```python
from build123d import *

# Parameters (mm, degrees)
BOSS_EXTRUDE1_DEPTH = 4.064
CUT_EXTRUDE1_DEPTH  = 5.08


with BuildPart() as part:
    # Sketch1 → Boss-Extrude1 (new body)
    with BuildSketch(Plane.XY):
        Polygon((-223.0755, -19.05), (-219.0115, -19.05), (-219.0115, -31.75), (-223.0755, -31.75), (-223.0755, -95.25), (-219.0115, -95.25), (-219.0115, -107.95), (-223.0755, -107.95), (-223.0755, -120.65), (223.0755, -120.65), (223.0755, -107.95), (219.0115, -107.95), (219.0115, -95.25), (223.0755, -95.25), (223.0755, -31.75), (219.0115, -31.75), (219.0115, -19.05), (223.0755, -19.05), (223.0755, 0), (172.2755, 0), (172.2755, 4.064), (146.8755, 4.064), (146.8755, 0), (-146.8755, 0), (-146.8755, 4.064), (-172.2755, 4.064), (-172.2755, 0), (-223.0755, 0), align=None)
    extrude(amount=BOSS_EXTRUDE1_DEPTH)

    # Sketch2 → Cut-Extrude1 (cut)
    with BuildSketch(Plane.XY.offset(4.064)):
        with BuildLine():
            Line((-105.7275, -25.4), (105.7275, -25.4))
            ThreePointArc((105.7275, -25.4), (114.707756121, -29.119743879), (118.4275, -38.1))
            Line((118.4275, -38.1), (118.4275, -82.55))
            ThreePointArc((118.4275, -82.55), (114.707756121, -91.530256121), (105.7275, -95.25))
            Line((105.7275, -95.25), (-105.7275, -95.25))
            ThreePointArc((-105.7275, -95.25), (-114.707756121, -91.530256121), (-118.4275, -82.55))
            Line((-118.4275, -82.55), (-118.4275, -38.1))
            ThreePointArc((-118.4275, -38.1), (-114.707756121, -29.119743879), (-105.7275, -25.4))
        make_face()
        with BuildLine():
            Line((137.88887808, -72.091607461), (157.460892539, -91.66362192))
            ThreePointArc((157.460892539, -91.66362192), (160.154969375, -91.66362192), (160.154969375, -88.969545084))
            Line((160.154969375, -88.969545084), (140.582954916, -69.397530625))
            ThreePointArc((140.582954916, -69.397530625), (137.88887808, -69.397530625), (137.88887808, -72.091607461))
        make_face()
        with BuildLine():
            Line((175.064666479, -90.408858006), (139.143641994, -54.487833521))
            ThreePointArc((139.143641994, -54.487833521), (136.449565158, -54.487833521), (136.449565158, -57.181910358))
            Line((136.449565158, -57.181910358), (172.370589642, -93.102934842))
            ThreePointArc((172.370589642, -93.102934842), (175.064666479, -93.102934842), (175.064666479, -90.408858006))
        make_face()
        with BuildLine():
            Line((139.728723609, -46.990684627), (182.561815373, -89.823776391))
            ThreePointArc((182.561815373, -89.823776391), (185.255892209, -89.823776391), (185.255892209, -87.129699554))
            Line((185.255892209, -87.129699554), (142.422800446, -44.296607791))
            ThreePointArc((142.422800446, -44.296607791), (139.728723609, -44.296607791), (139.728723609, -46.990684627))
        make_face()
        with BuildLine():
            Line((145.429821279, -39.221398115), (190.331101885, -84.122678721))
            ThreePointArc((190.331101885, -84.122678721), (193.025178721, -84.122678721), (193.025178721, -81.428601885))
            Line((193.025178721, -81.428601885), (148.123898115, -36.527321279))
            ThreePointArc((148.123898115, -36.527321279), (145.429821279, -36.527321279), (145.429821279, -39.221398115))
        make_face()
        with BuildLine():
            Line((153.199107791, -33.520300446), (196.032199554, -76.353392209))
            ThreePointArc((196.032199554, -76.353392209), (198.726276391, -76.353392209), (198.726276391, -73.659315373))
            Line((198.726276391, -73.659315373), (155.893184627, -30.826223609))
            ThreePointArc((155.893184627, -30.826223609), (153.199107791, -30.826223609), (153.199107791, -33.520300446))
        make_face()
        with BuildLine():
            Line((202.005434842, -63.468089642), (166.084410358, -27.547065158))
            ThreePointArc((166.084410358, -27.547065158), (163.390333521, -27.547065158), (163.390333521, -30.241141994))
            Line((163.390333521, -30.241141994), (199.311358006, -66.162166479))
            ThreePointArc((199.311358006, -66.162166479), (202.005434842, -66.162166479), (202.005434842, -63.468089642))
        make_face()
        with BuildLine():
            Line((178.300030625, -31.680454916), (197.872045084, -51.252469375))
            ThreePointArc((197.872045084, -51.252469375), (200.56612192, -51.252469375), (200.56612192, -48.558392539))
            Line((200.56612192, -48.558392539), (180.994107461, -28.98637808))
            ThreePointArc((180.994107461, -28.98637808), (178.300030625, -28.98637808), (178.300030625, -31.680454916))
        make_face()
    extrude(amount=-CUT_EXTRUDE1_DEPTH, mode=Mode.SUBTRACT)


solid = part.part
```
CAD build for the part. Positions are in the model's coordinates, mm. A direction names the side the tool comes from. Round coordinates to 2 decimals unless told otherwise and drop trailing zeros. Write each loop counter-clockwise with the first axis right and the second up, starting at its lowest first coordinate (ties: lowest second). Pieces come first, ordered by that corner, then holes. Notation, with made-up numbers: (55.5, 14) - (105.5, 14) arc R24 ccw to (105.5, 29) - close; hole circle Ø1 at (5.25, -17.75). An arc over 180 degrees is marked (long way). Return JSON: item names as keys, results as strings. Group by question number.
Item 1: Band-saw the part on B-B on z = 2.6. State how many separate pieces and enclosed holes the cut face has, plus the area to 3 significant figures.
Item 2: Band-saw the part on A-A on x = 21.5. List the corners of the cut face in (y, z).
Item 3: 3-axis set-ups, long thin cutter, end or side, ignore diameter. For faces 3 (the face through (-3, -99, 0)), 4 (the face through (147.5, -81.7, 2.1)): which of +Z, -Z, +X, -X, +Y, -Y reach the whole face in a straight line?
Item 4: Probe probe 1 along Y at (x, z) = (12, 2.4); probe 2 along X at (y, z) = (-37.5, 2.75); probe 3 along X at (y, z) = (-35, 1.5). List the from-to ranges inside material, lowest first.
Item 5: Mould opens along X. For faces 1 (the face through (150.506, -79.321, 2.06)), 2 (the face through (-3, -99, 4.064)) say: +X half, -X half, draft (parallel to the pull), parting line (faces both ways), or undercut.
Item 6: Flat gauge pins, fed straight in: pin 1 Ø2 at (y, z) = (-26, 1.5) entering from +X; pin 2 Ø1.2 at (x, z) = (-195, 1.5) entering from +Y; pin 3 Ø1.5 at (y, z) = (-107, 3) entering from -X. Where does each tip first touch, or does it go through?
Resolved:
{
 "1": {"separate pieces": "1", "enclosed holes": "8", "area": "36,000 mm²"},
 "2": {"outline": "(-120.65, 0) - (-95.25, 0) - (-95.25, 4.06) - (-120.65, 4.06) - close; (-25.4, 0) - (0, 0) - (0, 4.06) - (-25.4, 4.06) - close"},
 "3": {"face 3": "-Z, +X, -X, +Y, -Y", "face 4": "+Z, -Z"},
 "4": {"probe 1": "y = -120.65 to -95.25, -25.4 to 0", "probe 2": "x = -223.08 to -118.41, 118.41 to 144.91, 149.1 to 157.18, 162.57 to 170.65, 176.04 to 184.12, 189.51 to 223.08", "probe 3": "x = -223.08 to -118.04, 118.04 to 154.68, 160.07 to 168.15, 173.54 to 181.62, 187.01 to 223.08"},
 "5": {"face 1": "undercut", "face 2": "draft"},
 "6": {"pin 1": "stops at x = 219.01", "pin 2": "stops at y = 0", "pin 3": "stops at x = -219.01"}
}
